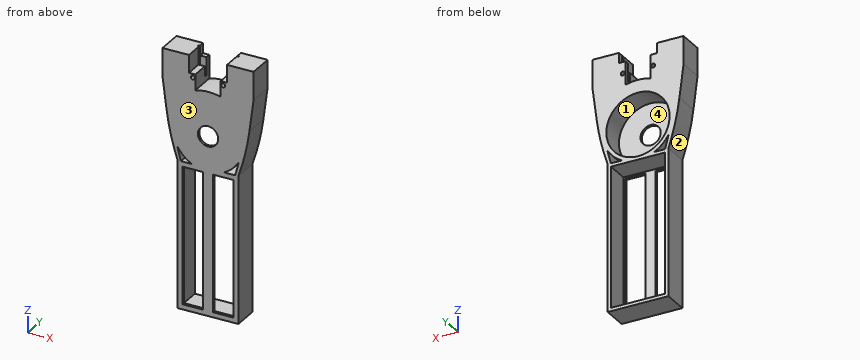
```python
from build123d import *

# Parameters (mm, degrees)
RESSALTO_EXTRUS_O1_DEPTH   = 11
RESSALTO_EXTRUS_O1_2_DEPTH = 11
RESSALTO_EXTRUS_O2_START   = -5
ESBO_O3_R                  = 12.5
ESBO_O3_W                  = 8
ESBO_O3_H                  = 54
RESSALTO_EXTRUS_O2_DEPTH   = 10
ESBO_O4_W                  = 21.4
ESBO_O4_H                  = 55.4
CORTE_EXTRUS_O1_DEPTH      = 9
CORTE_EXTRUS_O2_REACH      = 12
ESBO_O5_W                  = 2.5
ESBO_O5_H                  = 7
ESBO_O6_R                  = 0.8
ESBO_O6_W                  = 15
ESBO_O6_H                  = 4
CORTE_EXTRUS_O3_DEPTH      = 11
CORTE_EXTRUS_O4_DEPTH      = 1
CORTE_EXTRUS_O4_DEPTH_BACK = 11
ESBO_O10_R                 = 12.5
ESBO_O10_R_2               = 4
RESSALTO_EXTRUS_O3_DEPTH   = 1


with BuildPart() as part:
    # Esbo_o1 → Ressalto-extrus_o1 (new body)
    with BuildSketch(Plane.XY):
        Polygon((-5, 1.8), (-5, -5), (-14.1, -5), (-14.1, 5), (-5, 5), (-5, 3), (-7.5, 3), (-8.1, 2.4), (-7.5, 1.8), align=None)
    extrude(amount=RESSALTO_EXTRUS_O1_DEPTH)



with BuildPart() as body_2:
    # Esbo_o1 → Ressalto-extrus_o1 2 (new body)
    with BuildSketch(Plane.XY):
        Polygon((7.5, 1.8), (5, 1.8), (5, -5), (14.1, -5), (14.1, 5), (5, 5), (5, 3), (7.5, 3), (8.1, 2.4), align=None)
    extrude(amount=RESSALTO_EXTRUS_O1_2_DEPTH)


with BuildPart() as part_1:
    add(part.part)

    add(body_2.part)  # Ressalto-extrus_o2 merges body 2
    # Esbo_o3 → Ressalto-extrus_o2 (add, through all)
    with BuildSketch(Plane(origin=(0, 0, 0), x_dir=(1, 0, 0), z_dir=(0, 1, 0)).offset(RESSALTO_EXTRUS_O2_START)):
        with BuildLine():
            Line((-14.1, -11), (-14.1, 0))
            Line((-14.1, 0), (-5, 0))
            Line((-5, 0), (-5, 2.229490169))
            ThreePointArc((-5, 2.229490169), (0, 1.5), (5, 2.229490169))
            Line((5, 2.229490169), (5, 0))
            Line((5, 0), (14.1, 0))
            Line((14.1, 0), (14.1, -11))
            Line((14.1, -11), (18, -11))
            Line((18, -11), (18, 0))
            Line((18, 0), (16.353425267, 12.769792778))
            ThreePointArc((16.353425267, 12.769792778), (14.646005419, 22.243973189), (12, 31.5))
            Line((12, 31.5), (12, 89.5))
            Line((12, 89.5), (-12, 89.5))
            Line((-12, 89.5), (-12, 31.5))
            ThreePointArc((-12, 31.5), (-14.646005419, 22.243973189), (-16.353425267, 12.769792778))
            Line((-16.353425267, 12.769792778), (-18, 0))
            Line((-18, 0), (-18, -11))
            Line((-18, -11), (-14.1, -11))
        make_face()
        with Locations((0, 19)):
            Circle(ESBO_O3_R, mode=Mode.SUBTRACT)
        with Locations((-6, 60.5)):
            Rectangle(ESBO_O3_W, ESBO_O3_H, mode=Mode.SUBTRACT)
        with Locations((6, 60.5)):
            Rectangle(ESBO_O3_W, ESBO_O3_H, mode=Mode.SUBTRACT)
    extrude(amount=RESSALTO_EXTRUS_O2_DEPTH)

    # Esbo_o4 → Corte-extrus_o1 (cut)
    with BuildSketch(Plane(origin=(0, 5, 0), x_dir=(1, 0, 0), z_dir=(0, 1, 0))):
        with Locations((0, 60.5)):
            Rectangle(ESBO_O4_W, ESBO_O4_H)
    extrude(amount=-CORTE_EXTRUS_O1_DEPTH, mode=Mode.SUBTRACT)

    # Esbo_o5 → Corte-extrus_o2 (cut, up to next)
    with BuildSketch(Plane.XZ.offset(5), mode=Mode.PRIVATE) as corte_extrus_o2_sk1:
        with Locations((-6.25, 7.5)):
            Rectangle(ESBO_O5_W, ESBO_O5_H)
    corte_extrus_o2_tool1 = extrude(corte_extrus_o2_sk1.sketch, amount=-CORTE_EXTRUS_O2_REACH, mode=Mode.PRIVATE) & part_1.part
    add(corte_extrus_o2_tool1.solids().sort_by_distance((-6.25, -5, 7.5))[0], mode=Mode.SUBTRACT)
    # Esbo_o5 → Corte-extrus_o2 (cut, up to next)
    with BuildSketch(Plane.XZ.offset(5), mode=Mode.PRIVATE) as corte_extrus_o2_sk2:
        with Locations((6.25, 7.5)):
            Rectangle(ESBO_O5_W, ESBO_O5_H)
    corte_extrus_o2_tool2 = extrude(corte_extrus_o2_sk2.sketch, amount=-CORTE_EXTRUS_O2_REACH, mode=Mode.PRIVATE) & part_1.part
    add(corte_extrus_o2_tool2.solids().sort_by_distance((6.25, -5, 7.5))[0], mode=Mode.SUBTRACT)

    # Esbo_o6 → Corte-extrus_o3 (cut, through all)
    with BuildSketch(Plane(origin=(0, 5, 0), x_dir=(1, 0, 0), z_dir=(0, 1, 0))):
        with Locations((-6, -2.5)):
            Circle(ESBO_O6_R)
        with Locations((6, -2.5)):
            Circle(ESBO_O6_R)
        with Locations((0, -9)):
            Rectangle(ESBO_O6_W, ESBO_O6_H)
    extrude(amount=-CORTE_EXTRUS_O3_DEPTH, mode=Mode.SUBTRACT)

    # Esbo_o9 → Corte-extrus_o4 (cut, two sides)
    with BuildSketch(Plane(origin=(0, 5, 0), x_dir=(1, 0, 0), z_dir=(0, 1, 0))) as corte_extrus_o4_sk:
        with BuildLine():
            Line((6.304760106, 31.5), (10.7, 31.5))
            ThreePointArc((10.7, 31.5), (11.444665091, 28.788992569), (12.093349717, 26.053431266))
            ThreePointArc((12.093349717, 26.053431266), (9.593690062, 29.196132158), (6.304760106, 31.5))
        make_face()
        with BuildLine():
            Line((-6.304760106, 31.5), (-10.7, 31.5))
            ThreePointArc((-10.7, 31.5), (-11.444665091, 28.788992569), (-12.093349717, 26.053431266))
            ThreePointArc((-12.093349717, 26.053431266), (-9.593690062, 29.196132158), (-6.304760106, 31.5))
        make_face()
    extrude(amount=CORTE_EXTRUS_O4_DEPTH, mode=Mode.SUBTRACT)
    extrude(corte_extrus_o4_sk.sketch, amount=-CORTE_EXTRUS_O4_DEPTH_BACK, mode=Mode.SUBTRACT)

    # Esbo_o10 → Ressalto-extrus_o3 (add)
    with BuildSketch(Plane.XZ.offset(5)):
        with Locations((0, -19)):
            Circle(ESBO_O10_R)
        with Locations((0, -19)):
            Circle(ESBO_O10_R_2, mode=Mode.SUBTRACT)
    extrude(amount=-RESSALTO_EXTRUS_O3_DEPTH)


solid = part_1.part
```
Geometry check sheet. Reference: the model listing, model coordinates, mm. Face numbers are marked on the shaded views. Give positions to 0.01 mm unless a question says otherwise; leave off trailing zeros. Order: outer loops, then holes, each group sorted by start corner. A loop starts at its lowest first (then second) coordinate and runs counter-clockwise, first axis right, second up. Notation, with made-up numbers: (-17.75, -37.75) - (20.25, -37.75) arc R13 ccw to (20.25, -31.75) - close; hole circle Ø7 at (51, 17.25). An arc over 180 degrees is marked (long way). Answer in a Markdown table with one row per item. Add a question column.
Q1. Cross-section at C-C, the plane y = -3. Count the separate pieces of the cut face and the enclosed holes in it, then the cut area to 3 significant figures.
Q2. Material ranges on probe 1 along X at (y, z) = (-3.25, 2.5); probe 2 along Z at (x, y) = (0, 0.25); probe 3 along X at (y, z) = (1.25, -61), recorded low to high. Write a range as from..to.
Q3. Gauge pin test, flat ends, axial feed: pin 1 (2 mm diameter, centred on x = 6, y = 4, fed in from +Z); pin 2 (4.5 mm diameter, centred on y = -1, z = -59, fed in from +X); pin 3 (1.1 mm diameter, centred on y = -4.5, z = -47.5, fed in from -X). Record the tip position at first contact, or that the pin passes through.
Q4. Cross-section at A-A, the plane z = -75.5. Enter the section's corners in (x, y).
Q5. Mould release check, pull along X, two halves, no side actions. Record for the marked faces 1, 2, 3 and 4: pulls with the +X half, pulls with the -X half, needs draft (parallel to the pull), parting line crosses it, or undercut.
Q6. Cross-section at B-B, the plane x = 0. Enter the section's corners in (y, z), then the cut area to 3 significant figures.
Q7. Cross-section at D-D, the plane z = -19. Enter the section's corners in (x, y), then the cut area to 3 significant figures.
Check values:
| question | item | result |
|---|---|---|
| 1 | separate pieces | 1 |
| 1 | enclosed holes | 6 |
| 1 | area | 909 mm^2 |
| 2 | probe 1 | x = -18..-6.8, -5.2..-5, 5..5.2, 6.8..18 |
| 2 | probe 2 | z = -89.5..-88.2, -32.8..-31.5, -6.5..-1.5 |
| 2 | probe 3 | x = -12..-10.7, 10.7..12 |
| 3 | pin 1 | stops at z = 7 |
| 3 | pin 2 | stops at x = 12 |
| 3 | pin 3 | stops at x = -12 |
| 4 | outline | (-12, -5) - (-10, -5) - (-10, -4) - (-10.7, -4) - (-10.7, 5) - (-12, 5) - close; (-2, -5) - (2, -5) - (2, -4) - (-2, -4) - close; (10, -5) - (12, -5) - (12, 5) - (10.7, 5) - (10.7, -4) - (10, -4) - close |
| 5 | face 1 | undercut |
| 5 | face 2 | pulls with the -X half |
| 5 | face 3 | needs draft |
| 5 | face 4 | undercut |
| 6 | outline | (-5, -89.5) - (5, -89.5) - (5, -88.2) - (-4, -88.2) - (-4, -32.8) - (5, -32.8) - (5, -31.5) - (-4, -31.5) - (-4, -23) - (-5, -23) - close; (-5, -15) - (-4, -15) - (-4, -6.5) - (5, -6.5) - (5, -1.5) - (-5, -1.5) - close |
| 6 | area | 148 mm^2 |
| 7 | outline | (-15.34, -5) - (-4, -5) - (-4, -4) - (-12.5, -4) - (-12.5, 5) - (-15.34, 5) - close; (4, -5) - (15.34, -5) - (15.34, 5) - (12.5, 5) - (12.5, -4) - (4, -4) - close |
| 7 | area | 73.8 mm^2 |
